Part model, mm, in its own coordinate system. Give positions to 0.01 mm unless a question says otherwise; leave off trailing zeros. Loops run counter-clockwise (first coordinate to the right, second up) from the corner with the lowest first, then second, coordinate; pieces in that order, holes last. Notation, with made-up numbers: (11, -8) -> (16, -8) arc R26 cw to (16, 10) -> close; hole circle Ø7 at (-33.5, -5.5). An arc over 180 degrees is marked (long way). Write item = value, one per line.
from build123d import *

# Parameters (mm, degrees)
F0_W     = 12
F0_H     = 3
F0_W_2   = 3
F0_H_2   = 20
F0_H_3   = 44
F0_H_4   = 6
F1_DEPTH = 1.5
F3_DEPTH = 1.5


# Not quite as in the source:
# - a feature of the source that left no trace in its solid (it failed there, or was rolled back) is left out


with BuildPart() as f1:
    # F0 (on Front) → F1 (new body, symmetric)
    with BuildSketch(Plane.XZ):
        with BuildLine():
            Line((-147.1994572369, 90.198807884), (-184.1994572369, 90.198807884))
            Line((-184.1994572369, 90.198807884), (-184.1994572369, 84.198807884))
            Line((-184.1994572369, 84.198807884), (-181.1994572369, 84.198807884))
            Line((-181.1994572369, 84.198807884), (-181.1994572369, 78.198807884))
            Line((-181.1994572369, 78.198807884), (-184.1994572369, 78.198807884))
            Line((-184.1994572369, 78.198807884), (-184.1994572369, 13.198807884))
            Line((-184.1994572369, 13.198807884), (-181.1994572369, 13.198807884))
            Line((-181.1994572369, 13.198807884), (-181.1994572369, -6.801192116))
            Line((-181.1994572369, -6.801192116), (-184.1994572369, -6.801192116))
            Line((-184.1994572369, -6.801192116), (-184.1994572369, -31.801192116))
            Line((-184.1994572369, -31.801192116), (-166.1994572369, -31.801192116))
            Line((-166.1994572369, -31.801192116), (-166.1994572369, -9.4251137796))
            ThreePointArc((-166.1994572369, -9.4251137796), (-165.6004708263, -4.5670615257), (-163.8393900667, 0))
            Line((-163.8393900667, 0), (-137.559524407, 49.1850895229))
            ThreePointArc((-137.559524407, 49.1850895229), (-135.7984436474, 53.7521510486), (-135.1994572369, 58.6102033025))
            Line((-135.1994572369, 58.6102033025), (-135.1994572369, 90.198807884))
            Line((-135.1994572369, 90.198807884), (-141.1994572369, 90.198807884))
            Line((-141.1994572369, 90.198807884), (-141.1994572369, 87.198807884))
            Line((-141.1994572369, 87.198807884), (-147.1994572369, 87.198807884))
            Line((-147.1994572369, 87.198807884), (-147.1994572369, 90.198807884))
        make_face()
        with Locations((-175.1994572369, -27.301192116)):
            Rectangle(F0_W, F0_H, mode=Mode.SUBTRACT)
        with Locations((-167.6994572369, 14.198807884)):
            Rectangle(F0_W_2, F0_H_2, mode=Mode.SUBTRACT)
        with Locations((-175.1994572369, 50.198807884)):
            Rectangle(F0_W, F0_H_3, mode=Mode.SUBTRACT)
        with Locations((-167.6994572369, 81.198807884)):
            Rectangle(F0_W_2, F0_H_4, mode=Mode.SUBTRACT)
    extrude(amount=F1_DEPTH, both=True)

    # F0 (on Front) → F3 (cut, symmetric)
    with BuildSketch(Plane.XZ):
        with Locations((-175.1994572369, -27.301192116)):
            Rectangle(F0_W, F0_H)
    extrude(amount=F3_DEPTH, both=True, mode=Mode.SUBTRACT)


solid = f1.part
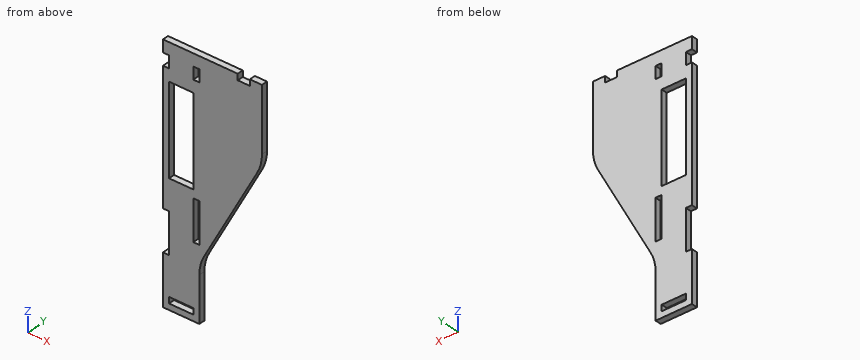
1) Drill centre lines: line 1 along Z through (x, y) = (-179.5, -0.1); line 2 along X through (y, z) = (1.05, 71.5); line 3 along X through (y, z) = (0.65, -19). Where is each one in solid material? Low to high. Write a range as [from, to].
Resolved:
line_1 = [-31.8, -28.8], [-25.8, 28.2], [72.2, 90.2]
line_2 = [-184.2, -181.2], [-169.2, -135.2]
line_3 = [-184.2, -166.2]
2) Drop flat-ended pins along their axis: P1, Ø1.5, axis at y = -0.5, z = 12, coming from the -X side; P2, Ø0.9, axis at y = 0, z = -20.5, coming from the +X side; P3, Ø0.9, axis at x = -145, y = 0.5, coming from the +Z side. Give the stop position or say it passes through.
Resolved:
P1 = -181.2
P2 = -166.2
P3 = 87.2
3) Slice it at A-A, the plane y = -0.2. Count the separate pieces of the cut face and the enclosed holes in it, and give its area (3 significant figures).
Resolved:
separate_pieces = 1
enclosed_holes = 4
area = 3,490 mm²
4) Slice it at B-B, the plane x = -145. List the corners of the cut face in (y, z).
Resolved:
outline = (-1.5, 35.26) -> (1.5, 35.26) -> (1.5, 87.2) -> (-1.5, 87.2) -> close
5) Slice it at C-C, the plane z = -20. List the corners of the cut face in (x, y).
Resolved:
outline = (-184.2, -1.5) -> (-166.2, -1.5) -> (-166.2, 1.5) -> (-184.2, 1.5) -> close
